Can you work these out from the model? Positions are in its coordinate system, mm. Face numbers are marked on the shaded views. A direction names the side the tool comes from. Coordinates: 2 decimals unless noted, no trailing zeros. Write each loop counter-clockwise with the first axis right and the second up, starting at its lowest first coordinate (ties: lowest second). Pieces come first, ordered by that corner, then holes. Notation, with made-up numbers: M 47.25,-26.5 L 81.25,-26.5 A18 ccw 81.25,2.5 Z; hole C -27,17.25 d1. An arc over 180 degrees is marked long. Answer as a JSON object with one key per item and string values. Group by question number.
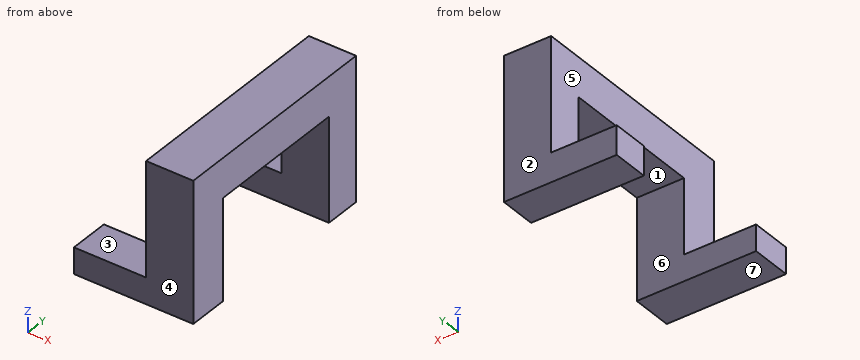
from build123d import *

# Parameters (mm, degrees)
F1_DEPTH = 18.288
F2_W     = 14.2342057079
F2_H     = 11.2496130168
F3_DEPTH = 25.4
F4_W     = 12.39753142
F4_H     = 10.101692751
F5_DEPTH = 27.94
F6_DEPTH = 3.302


with BuildPart() as f1:
    # F0 (on Right) → F1 (new body)
    with BuildSketch(Plane.YZ):
        Polygon((-44.8836572468, 44.0801158547), (-44.8836572468, -10.101692751), (-32.4861258268, -10.101692751), (-32.4861258268, 28.9275757968), (26.2873601168, 28.9275757968), (26.2873601168, -11.2496130168), (40.5215658247, -11.2496130168), (40.5215658247, 44.0801158547), align=None)
    extrude(amount=-F1_DEPTH)

    # F2 (on face) → F3 (join)
    with BuildSketch(Plane(origin=(-18.288, 0, 0), x_dir=(0, -1, 0), z_dir=(-1, 0, 0))):
        with Locations((-33.4044629708, -5.6248065084)):
            Rectangle(F2_W, F2_H)
    extrude(amount=F3_DEPTH)

    # F4 (on face) → F5 (join)
    with BuildSketch(Plane(origin=(-18.288, 0, 0), x_dir=(0, -1, 0), z_dir=(-1, 0, 0))):
        with Locations((38.6848915368, -5.0508463755)):
            Rectangle(F4_W, F4_H)
    extrude(amount=F5_DEPTH)

    # F6 (add): a face of the model
    f6_faces = [f1.faces().sort_by_distance(p)[0] for p in [
        (-15.6938687201, -32.4861258268, 5.3143038172),
    ]]
    extrude(f6_faces, amount=F6_DEPTH)


solid = f1.part
Q1. If we section it at A-A on x = -34: List the corners of the cut face in (y, z) for me, and give its area (3 significant figures).
Q2. We'd pull the mould along Y, two halves only. Please class the marked faces 1, 2, 3 and 4: pulls with the +Y half, pulls with the -Y half, needs draft (parallel to the pull), parting line crosses it, or undercut.
Q3. If we section it at D-D on y = -33: List the corners of the cut face in (x, z) for me.
Q4. If we section it at C-C on x = -5: List the corners of the cut face in (y, z) for me, and give its area (3 significant figures).
Q5. Please list where these lines run through material, in increasing order: L1, parallel to Y at x = -3.5, z = 9.5; L2, parallel to Z at x = -6.5, y = -33; L3, parallel to X at y = -35.5, z = 13.5.
Q6. If we section it at B-B on z = 20.5: List the corners of the cut face in (x, y) for me, and give its area (3 significant figures).
Q7. Will these pins go through, and if not, where does the flat tip stop? pin 1 (4.5 mm diameter, centred on x = -29.5, y = -39.5, fed in from -Z); pin 2 (15.5 mm diameter, centred on x = -36.5, y = 30.5, fed in from +Z); pin 3 (10 mm diameter, centred on y = 1, z = 32.5, fed in from +X); pin 4 (20 mm diameter, centred on x = -6, y = -10.5, fed in from -Z).
Q8. On a 3-axis mill with a long thin cutter (end or side, diameter ignored), from which of +Z, -Z, +X, -X, +Y, -Y can I reach the whole of each face in a straight line? I mean the marked faces 5, 6 and 7. Say none if no direction works.
Reply:
{
 "1": {"outline": "M -44.88,-10.1 L -29.18,-10.1 L -29.18,0 L -44.88,0 Z; M 26.29,-11.25 L 40.52,-11.25 L 40.52,0 L 26.29,0 Z", "area": "319 mm^2"},
 "2": {"face 1": "undercut", "face 2": "pulls with the +Y half", "face 3": "needs draft", "face 4": "pulls with the -Y half"},
 "3": {"outline": "M -46.23,-10.1 L 0,-10.1 L 0,44.08 L -18.29,44.08 L -18.29,0 L -46.23,0 Z"},
 "4": {"outline": "M -44.88,-10.1 L -29.18,-10.1 L -29.18,28.93 L 26.29,28.93 L 26.29,-11.25 L 40.52,-11.25 L 40.52,44.08 L -44.88,44.08 Z", "area": "2,480 mm^2"},
 "5": {"L1": "-44.88 to -29.18, 26.29 to 40.52", "L2": "-10.1 to 44.08", "L3": "-18.29 to 0"},
 "6": {"outline": "M -18.29,-44.88 L 0,-44.88 L 0,-29.18 L -18.29,-29.18 Z; M -18.29,26.29 L 0,26.29 L 0,40.52 L -18.29,40.52 Z", "area": "547 mm^2"},
 "7": {"pin 1": "z = -10.1", "pin 2": "z = 0", "pin 3": "x = 0", "pin 4": "z = 28.93"},
 "8": {"face 5": "+Z, -X, +Y, -Y", "face 6": "-Z, +X, -X", "face 7": "-Z, +X, -X, -Y"}
}
